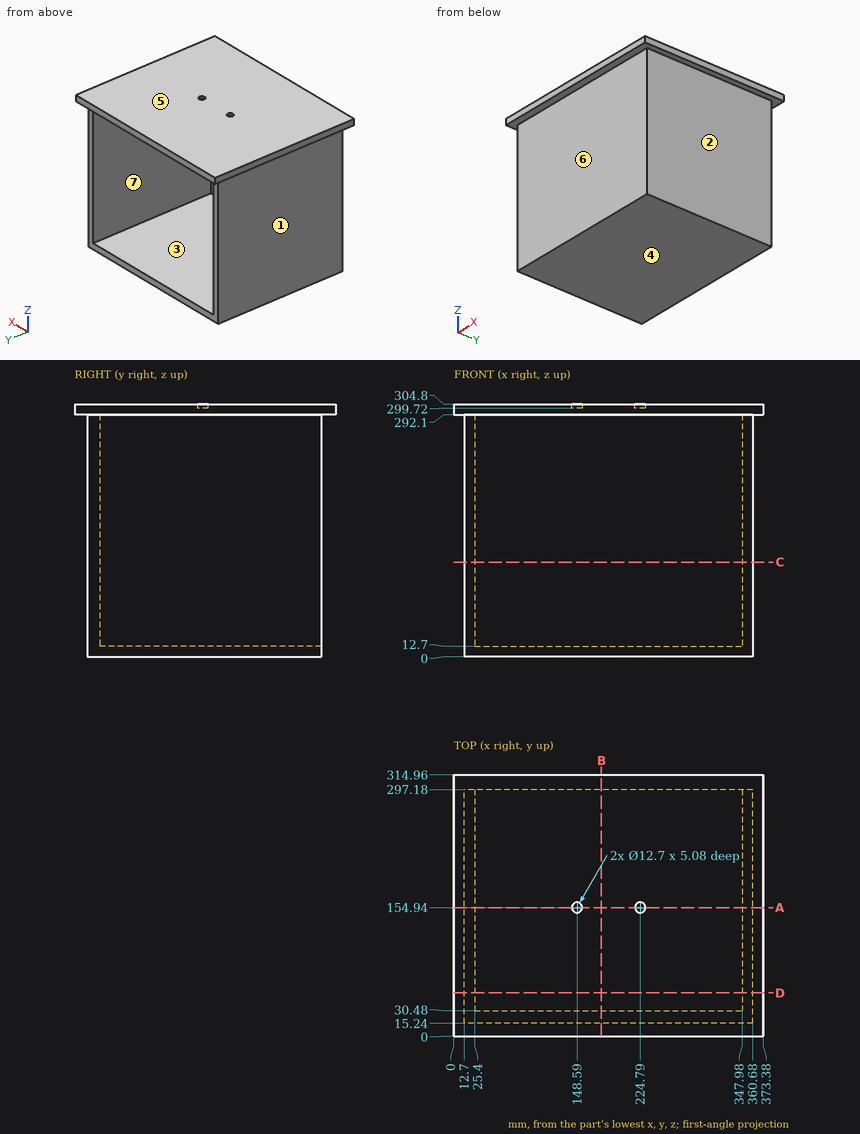
Here's the drawing with two shaded views (mm, measured from the low corner). I have some questions. A direction names the side the tool comes from. Give positions to 0.01 mm unless a question says otherwise; leave off trailing zeros. Loops run counter-clockwise (first coordinate to the right, second up) from the corner with the lowest first, then second, coordinate; pieces in that order, holes last. Notation, with made-up numbers: M 33.25,70 L 51.25,70 A26 ccw 51.25,102 Z; hole C 22.25,37.25 d7. An arc over 180 degrees is marked long. One line per item, written item: value.
1) I'm going to push flat-ended pins straight in: pin 1 (1 mm diameter, centred on x = 147, z = 212.5, fed in from -Y); pin 2 (10 mm diameter, centred on x = 147, y = 157, fed in from +Z); pin 3 (5 mm diameter, centred on x = 79, z = 54, fed in from +Y); pin 4 (6.5 mm diameter, centred on x = 223.5, y = 156, fed in from +Z). Where does each tip first touch, or does it pass through?
Geometry check:
pin 1: stops at y = 15.24
pin 2: stops at z = 304.8
pin 3: stops at y = 30.48
pin 4: stops at z = 299.72
2) Imagine slicing it at B-B on x = 178. Write out the boundary of the cut face in (y, z), and give its area (3 significant figures).
Geometry check:
outline: M 0,292.1 L 15.24,292.1 L 15.24,0 L 297.18,0 L 297.18,12.7 L 30.48,12.7 L 30.48,292.1 L 314.96,292.1 L 314.96,304.8 L 0,304.8 Z
area: 11,800 mm²
3) Please list where these lines run through material, in increasing order: line 1 (X direction, y = 154, z = 303); line 2 (Z direction, x = 27, y = 102); line 3 (X direction, y = 271, z = 289.5).
Geometry check:
line 1: x = 0 to 142.31, 154.87 to 218.51, 231.07 to 373.38
line 2: z = 0 to 12.7, 292.1 to 304.8
line 3: x = 12.7 to 25.4, 347.98 to 360.68
4) Thinking about a two-plate mould opening in X: for the marked faces 1, 2, 3 and 4, which applies, +X half, -X half, draft (parallel to the pull), parting line (faces both ways), or undercut?
Geometry check:
face 1: -X half
face 2: +X half
face 3: undercut
face 4: draft
5) Imagine slicing it at C-C on z = 114. Write out the boundary of the cut face in (x, y).
Geometry check:
outline: M 12.7,15.24 L 360.68,15.24 L 360.68,297.18 L 347.98,297.18 L 347.98,30.48 L 25.4,30.48 L 25.4,297.18 L 12.7,297.18 Z
6) On a 3-axis mill with a long thin cutter (end or side, diameter ignored), from which of +Z, -Z, +X, -X, +Y, -Y can I reach the whole of each face in a straight line? I mean the marked faces 5, 6 and 7. Say none if no direction works.
Geometry check:
face 5: +Z, +X, -X, +Y, -Y
face 6: -Z, +X, -X, -Y
face 7: +Y
7) Imagine slicing it at D-D on y = 52. Write out the boundary of the cut face in (x, z).
Geometry check:
outline: M 0,292.1 L 12.7,292.1 L 12.7,0 L 360.68,0 L 360.68,292.1 L 373.38,292.1 L 373.38,304.8 L 0,304.8 Z; hole M 25.4,12.7 L 347.98,12.7 L 347.98,292.1 L 25.4,292.1 Z
8) Imagine slicing it at A-A on y = 154.94. Write out the boundary of the cut face in (x, z), and give its area (3 significant figures).
Geometry check:
outline: M 0,292.1 L 12.7,292.1 L 12.7,0 L 360.68,0 L 360.68,292.1 L 373.38,292.1 L 373.38,304.8 L 231.14,304.8 L 231.14,299.72 L 218.44,299.72 L 218.44,304.8 L 154.94,304.8 L 154.94,299.72 L 142.24,299.72 L 142.24,304.8 L 0,304.8 Z; hole M 25.4,12.7 L 347.98,12.7 L 347.98,292.1 L 25.4,292.1 Z
area: 16,100 mm²
